from build123d import *

# Parameters (mm, degrees)
BOSS_EXTRUDE1_DEPTH     = 5
SKETCH5_R               = 17.5
BOSS_EXTRUDE2_DEPTH     = 2.5
CUT_EXTRUDE2_DEPTH      = 1
CUT_EXTRUDE2_DEPTH_BACK = 8.5


with BuildPart() as part:
    # Sketch1 → Boss-Extrude1 (new body)
    with BuildSketch(Plane(origin=(0, 0, 0), x_dir=(1, 0, 0), z_dir=(0, 1, 0))):
        with BuildLine():
            Line((-1.5, 24.494818027), (-3.75, 25.728146066))
            Line((-3.75, 25.728146066), (-4.75, 28.608346684))
            Line((-4.75, 28.608346684), (-5.5, 29.491524206))
            ThreePointArc((-5.5, 29.491524206), (-6.518225952, 29.283318296), (-7.528629065, 29.039968051))
            ThreePointArc((-7.528629065, 29.039968051), (-7.764571353, 28.977774789), (-8, 28.91366459))
            ThreePointArc((-8, 28.91366459), (-8.996709886, 28.619210528), (-9.982622382, 28.290409159))
            Line((-9.982622382, 28.290409159), (-10.190552674, 27.150554989))
            Line((-10.190552674, 27.150554989), (-9.616477769, 24.156228086))
            Line((-9.616477769, 24.156228086), (-10.948370908, 21.963134673))
            Line((-10.948370908, 21.963134673), (-10.700961894, 21.534609691))
            Line((-10.700961894, 21.534609691), (-13.299038106, 20.034609691))
            Line((-13.299038106, 20.034609691), (-13.546447119, 20.463134673))
            Line((-13.546447119, 20.463134673), (-16.111668297, 20.406228086))
            Line((-16.111668297, 20.406228086), (-18.41779401, 22.400554989))
            Line((-18.41779401, 22.400554989), (-19.508901824, 22.790409159))
            ThreePointArc((-19.508901824, 22.790409159), (-20.28660841, 22.100984575), (-21.039968051, 21.385035525))
            ThreePointArc((-21.039968051, 21.385035525), (-21.213203436, 21.213203436), (-21.385035525, 21.039968051))
            ThreePointArc((-21.385035525, 21.039968051), (-22.100984575, 20.28660841), (-22.790409159, 19.508901824))
            Line((-22.790409159, 19.508901824), (-22.400554989, 18.41779401))
            Line((-22.400554989, 18.41779401), (-20.406228086, 16.111668297))
            Line((-20.406228086, 16.111668297), (-20.463134673, 13.546447119))
            Line((-20.463134673, 13.546447119), (-20.034609691, 13.299038106))
            Line((-20.034609691, 13.299038106), (-21.534609691, 10.700961894))
            Line((-21.534609691, 10.700961894), (-21.963134673, 10.948370908))
            Line((-21.963134673, 10.948370908), (-24.156228086, 9.616477769))
            Line((-24.156228086, 9.616477769), (-27.150554989, 10.190552674))
            Line((-27.150554989, 10.190552674), (-28.290409159, 9.982622382))
            ThreePointArc((-28.290409159, 9.982622382), (-28.619210528, 8.996709886), (-28.91366459, 8))
            ThreePointArc((-28.91366459, 8), (-28.977774789, 7.764571353), (-29.039968051, 7.528629065))
            ThreePointArc((-29.039968051, 7.528629065), (-29.283318296, 6.518225952), (-29.491524206, 5.5))
            Line((-29.491524206, 5.5), (-28.608346684, 4.75))
            Line((-28.608346684, 4.75), (-25.728146066, 3.75))
            Line((-25.728146066, 3.75), (-24.494818027, 1.5))
            Line((-24.494818027, 1.5), (-24, 1.5))
            Line((-24, 1.5), (-24, -1.5))
            Line((-24, -1.5), (-24.494818027, -1.5))
            Line((-24.494818027, -1.5), (-25.728146066, -3.75))
            Line((-25.728146066, -3.75), (-28.608346684, -4.75))
            Line((-28.608346684, -4.75), (-29.491524206, -5.5))
            ThreePointArc((-29.491524206, -5.5), (-29.283318296, -6.518225952), (-29.039968051, -7.528629065))
            ThreePointArc((-29.039968051, -7.528629065), (-28.977774789, -7.764571353), (-28.91366459, -8))
            ThreePointArc((-28.91366459, -8), (-28.619210528, -8.996709886), (-28.290409159, -9.982622382))
            Line((-28.290409159, -9.982622382), (-27.150554989, -10.190552674))
            Line((-27.150554989, -10.190552674), (-24.156228086, -9.616477769))
            Line((-24.156228086, -9.616477769), (-21.963134673, -10.948370908))
            Line((-21.963134673, -10.948370908), (-21.534609691, -10.700961894))
            Line((-21.534609691, -10.700961894), (-20.034609691, -13.299038106))
            Line((-20.034609691, -13.299038106), (-20.463134673, -13.546447119))
            Line((-20.463134673, -13.546447119), (-20.406228086, -16.111668297))
            Line((-20.406228086, -16.111668297), (-22.400554989, -18.41779401))
            Line((-22.400554989, -18.41779401), (-22.790409159, -19.508901824))
            ThreePointArc((-22.790409159, -19.508901824), (-22.100984575, -20.28660841), (-21.385035525, -21.039968051))
            ThreePointArc((-21.385035525, -21.039968051), (-21.213203436, -21.213203436), (-21.039968051, -21.385035525))
            ThreePointArc((-21.039968051, -21.385035525), (-20.28660841, -22.100984575), (-19.508901824, -22.790409159))
            Line((-19.508901824, -22.790409159), (-18.41779401, -22.400554989))
            Line((-18.41779401, -22.400554989), (-16.111668297, -20.406228086))
            Line((-16.111668297, -20.406228086), (-13.546447119, -20.463134673))
            Line((-13.546447119, -20.463134673), (-13.299038106, -20.034609691))
            Line((-13.299038106, -20.034609691), (-10.700961894, -21.534609691))
            Line((-10.700961894, -21.534609691), (-10.948370908, -21.963134673))
            Line((-10.948370908, -21.963134673), (-9.616477769, -24.156228086))
            Line((-9.616477769, -24.156228086), (-10.190552674, -27.150554989))
            Line((-10.190552674, -27.150554989), (-9.982622382, -28.290409159))
            ThreePointArc((-9.982622382, -28.290409159), (-8.996709886, -28.619210528), (-8, -28.91366459))
            ThreePointArc((-8, -28.91366459), (-7.764571353, -28.977774789), (-7.528629065, -29.039968051))
            ThreePointArc((-7.528629065, -29.039968051), (-6.518225952, -29.283318296), (-5.5, -29.491524206))
            Line((-5.5, -29.491524206), (-4.75, -28.608346684))
            Line((-4.75, -28.608346684), (-3.75, -25.728146066))
            Line((-3.75, -25.728146066), (-1.5, -24.494818027))
            Line((-1.5, -24.494818027), (-1.5, -24))
            Line((-1.5, -24), (1.5, -24))
            Line((1.5, -24), (1.5, -24.494818027))
            Line((1.5, -24.494818027), (3.75, -25.728146066))
            Line((3.75, -25.728146066), (4.75, -28.608346684))
            Line((4.75, -28.608346684), (5.5, -29.491524206))
            ThreePointArc((5.5, -29.491524206), (6.518225952, -29.283318296), (7.528629065, -29.039968051))
            ThreePointArc((7.528629065, -29.039968051), (7.764571353, -28.977774789), (8, -28.91366459))
            ThreePointArc((8, -28.91366459), (8.996709886, -28.619210528), (9.982622382, -28.290409159))
            Line((9.982622382, -28.290409159), (10.190552674, -27.150554989))
            Line((10.190552674, -27.150554989), (9.616477769, -24.156228086))
            Line((9.616477769, -24.156228086), (10.948370908, -21.963134673))
            Line((10.948370908, -21.963134673), (10.700961894, -21.534609691))
            Line((10.700961894, -21.534609691), (13.299038106, -20.034609691))
            Line((13.299038106, -20.034609691), (13.546447119, -20.463134673))
            Line((13.546447119, -20.463134673), (16.111668297, -20.406228086))
            Line((16.111668297, -20.406228086), (18.41779401, -22.400554989))
            Line((18.41779401, -22.400554989), (19.508901824, -22.790409159))
            ThreePointArc((19.508901824, -22.790409159), (20.28660841, -22.100984575), (21.039968051, -21.385035525))
            ThreePointArc((21.039968051, -21.385035525), (21.213203436, -21.213203436), (21.385035525, -21.039968051))
            ThreePointArc((21.385035525, -21.039968051), (22.100984575, -20.28660841), (22.790409159, -19.508901824))
            Line((22.790409159, -19.508901824), (22.400554989, -18.41779401))
            Line((22.400554989, -18.41779401), (20.406228086, -16.111668297))
            Line((20.406228086, -16.111668297), (20.463134673, -13.546447119))
            Line((20.463134673, -13.546447119), (20.034609691, -13.299038106))
            Line((20.034609691, -13.299038106), (21.534609691, -10.700961894))
            Line((21.534609691, -10.700961894), (21.963134673, -10.948370908))
            Line((21.963134673, -10.948370908), (24.156228086, -9.616477769))
            Line((24.156228086, -9.616477769), (27.150554989, -10.190552674))
            Line((27.150554989, -10.190552674), (28.290409159, -9.982622382))
            ThreePointArc((28.290409159, -9.982622382), (28.619210528, -8.996709886), (28.91366459, -8))
            ThreePointArc((28.91366459, -8), (28.977774789, -7.764571353), (29.039968051, -7.528629065))
            ThreePointArc((29.039968051, -7.528629065), (29.283318296, -6.518225952), (29.491524206, -5.5))
            Line((29.491524206, -5.5), (28.608346684, -4.75))
            Line((28.608346684, -4.75), (25.728146066, -3.75))
            Line((25.728146066, -3.75), (24.494818027, -1.5))
            Line((24.494818027, -1.5), (24, -1.5))
            Line((24, -1.5), (24, 1.5))
            Line((24, 1.5), (24.494818027, 1.5))
            Line((24.494818027, 1.5), (25.728146066, 3.75))
            Line((25.728146066, 3.75), (28.608346684, 4.75))
            Line((28.608346684, 4.75), (29.491524206, 5.5))
            ThreePointArc((29.491524206, 5.5), (29.283318296, 6.518225952), (29.039968051, 7.528629065))
            ThreePointArc((29.039968051, 7.528629065), (28.977774789, 7.764571353), (28.91366459, 8))
            ThreePointArc((28.91366459, 8), (28.619210528, 8.996709886), (28.290409159, 9.982622382))
            Line((28.290409159, 9.982622382), (27.150554989, 10.190552674))
            Line((27.150554989, 10.190552674), (24.156228086, 9.616477769))
            Line((24.156228086, 9.616477769), (21.963134673, 10.948370908))
            Line((21.963134673, 10.948370908), (21.534609691, 10.700961894))
            Line((21.534609691, 10.700961894), (20.034609691, 13.299038106))
            Line((20.034609691, 13.299038106), (20.463134673, 13.546447119))
            Line((20.463134673, 13.546447119), (20.406228086, 16.111668297))
            Line((20.406228086, 16.111668297), (22.400554989, 18.41779401))
            Line((22.400554989, 18.41779401), (22.790409159, 19.508901824))
            ThreePointArc((22.790409159, 19.508901824), (22.100984575, 20.28660841), (21.385035525, 21.039968051))
            ThreePointArc((21.385035525, 21.039968051), (21.213203436, 21.213203436), (21.039968051, 21.385035525))
            ThreePointArc((21.039968051, 21.385035525), (20.28660841, 22.100984575), (19.508901824, 22.790409159))
            Line((19.508901824, 22.790409159), (18.41779401, 22.400554989))
            Line((18.41779401, 22.400554989), (16.111668297, 20.406228086))
            Line((16.111668297, 20.406228086), (13.546447119, 20.463134673))
            Line((13.546447119, 20.463134673), (13.299038106, 20.034609691))
            Line((13.299038106, 20.034609691), (10.700961894, 21.534609691))
            Line((10.700961894, 21.534609691), (10.948370908, 21.963134673))
            Line((10.948370908, 21.963134673), (9.616477769, 24.156228086))
            Line((9.616477769, 24.156228086), (10.190552674, 27.150554989))
            Line((10.190552674, 27.150554989), (9.982622382, 28.290409159))
            ThreePointArc((9.982622382, 28.290409159), (8.996709886, 28.619210528), (8, 28.91366459))
            ThreePointArc((8, 28.91366459), (7.764571353, 28.977774789), (7.528629065, 29.039968051))
            ThreePointArc((7.528629065, 29.039968051), (6.518225952, 29.283318296), (5.5, 29.491524206))
            Line((5.5, 29.491524206), (4.75, 28.608346684))
            Line((4.75, 28.608346684), (3.75, 25.728146066))
            Line((3.75, 25.728146066), (1.5, 24.494818027))
            Line((1.5, 24.494818027), (1.5, 24))
            Line((1.5, 24), (-1.5, 24))
            Line((-1.5, 24), (-1.5, 24.494818027))
        make_face()
    extrude(amount=BOSS_EXTRUDE1_DEPTH)

    # Sketch5 → Boss-Extrude2 (add)
    with BuildSketch(Plane.XZ):
        Circle(SKETCH5_R)
    extrude(amount=BOSS_EXTRUDE2_DEPTH)

    # Sketch6 → Cut-Extrude2 (cut, two sides)
    with BuildSketch(Plane.XZ.offset(2.5)) as cut_extrude2_sk:
        with BuildLine():
            ThreePointArc((4.125, 0), (3.82214204, 1.551404275), (2.958039892, 2.875))
            Line((2.958039892, 2.875), (-2.958039892, 2.875))
            ThreePointArc((-2.958039892, 2.875), (-1.551404275, -3.82214204), (4.125, 0))
        make_face()
    extrude(amount=CUT_EXTRUDE2_DEPTH, mode=Mode.SUBTRACT)
    extrude(cut_extrude2_sk.sketch, amount=-CUT_EXTRUDE2_DEPTH_BACK, mode=Mode.SUBTRACT)


solid = part.part
Check sheet for the modelled part. Datum: model origin and axes. Units: mm. A direction names the side the tool comes from. Round coordinates to 2 decimals unless told otherwise and drop trailing zeros. Order: outer loops, then holes, each group sorted by start corner. A loop starts at its lowest first (then second) coordinate and runs counter-clockwise, first axis right, second up.
Q1. Draft check along X on faces 6 (the face through (25.1, 2.5, -2.6)), 7 (the face through (25.674, 2.465, -9.908)), 8 (the face through (-21.417, 2.465, -17.281)). Enter one of: pulls with the +X half, pulls with the -X half, needs draft (parallel to the pull), parting line crosses it, or undercut.
Filled sheet:
face 6: pulls with the +X half
face 7: undercut
face 8: pulls with the -X half
Q2. Set-up check for faces 1 (the face through (4.257, 2.465, -27.188)), 2 (the face through (24, 2, 0)), 3 (the face through (-20.276, 2.465, -22.111)), 4 (the face through (17.25, 2.46, 21.39)), 5 (the face through (10.292, 2.465, -23.044)): record each of +Z, -Z, +X, -X, +Y, -Y from which the full face is reachable in a straight line by a thin tool's end or side.
Filled sheet:
face 1: -Z, +Y, -Y
face 2: +X, +Y, -Y
face 3: -Z, -X, +Y, -Y
face 4: +Z, +Y, -Y
face 5: +Y, -Y
Q3. Cross-section at A-A, the plane x = 0. Enter the section's corners in (y, z) (3 decimals).
Filled sheet:
outline: (-2.5, -17.5) - (0, -17.5) - (0, -24) - (5, -24) - (5, -4.125) - (-2.5, -4.125) - close; (-2.5, 2.875) - (5, 2.875) - (5, 24) - (0, 24) - (0, 17.5) - (-2.5, 17.5) - close
Q4. Cross-section at B-B, the plane x = 15. Enter the section's corners in (y, z), plus the area to 3 significant figures.
Filled sheet:
outline: (-2.5, -9.01) - (0, -9.01) - (0, -20.43) - (5, -20.43) - (5, 20.43) - (0, 20.43) - (0, 9.01) - (-2.5, 9.01) - close
area: 249 mm2
Q5. Depth check by flat-ended pin: P1, Ø1, axis at x = 2.5, y = 1.5, coming from the +Z side; P2, Ø1.5, axis at x = -0.5, y = 1.5, coming from the +Z side; P3, Ø3, axis at x = -0.5, y = 1, coming from the -Z side; P4, Ø3, axis at x = 6, y = 3.5, coming from the +Z side. Enter the tip coordinate at first touch or a pass-through.
Filled sheet:
P1: stops at z = 25.32
P2: stops at z = 24
P3: stops at z = -24.77
P4: stops at z = 29.49
Q6. Scan lines: L1, parallel to Z at x = 0, y = 2.5 (3 decimals); L2, parallel to X at y = 3.25, z = -20.5; L3, parallel to Z at x = 19.5, y = 3.5. Record each from-to range of solid material in increasing order.
Filled sheet:
L1: z = -24 to -4.125, 2.875 to 24
L2: x = -21.9 to -16.22, -12.49 to 12.49, 16.22 to 21.9
L3: z = -22.79 to 22.79
